Drawing for the job (mm, zero at the part's lowest x, y, z). A direction names the side the tool comes from. Coordinates: 2 decimals unless noted, no trailing zeros. Loops run counter-clockwise (first coordinate to the right, second up) from the corner with the lowest first, then second, coordinate; pieces in that order, holes last. Notation, with made-up numbers: (53, 24) -> (79, 24) arc R16 ccw to (79, 42) -> close; hole circle Ø9 at (-32, 68). An arc over 180 degrees is marked (long way). Write each question's results on one line, items separated by ' | '.
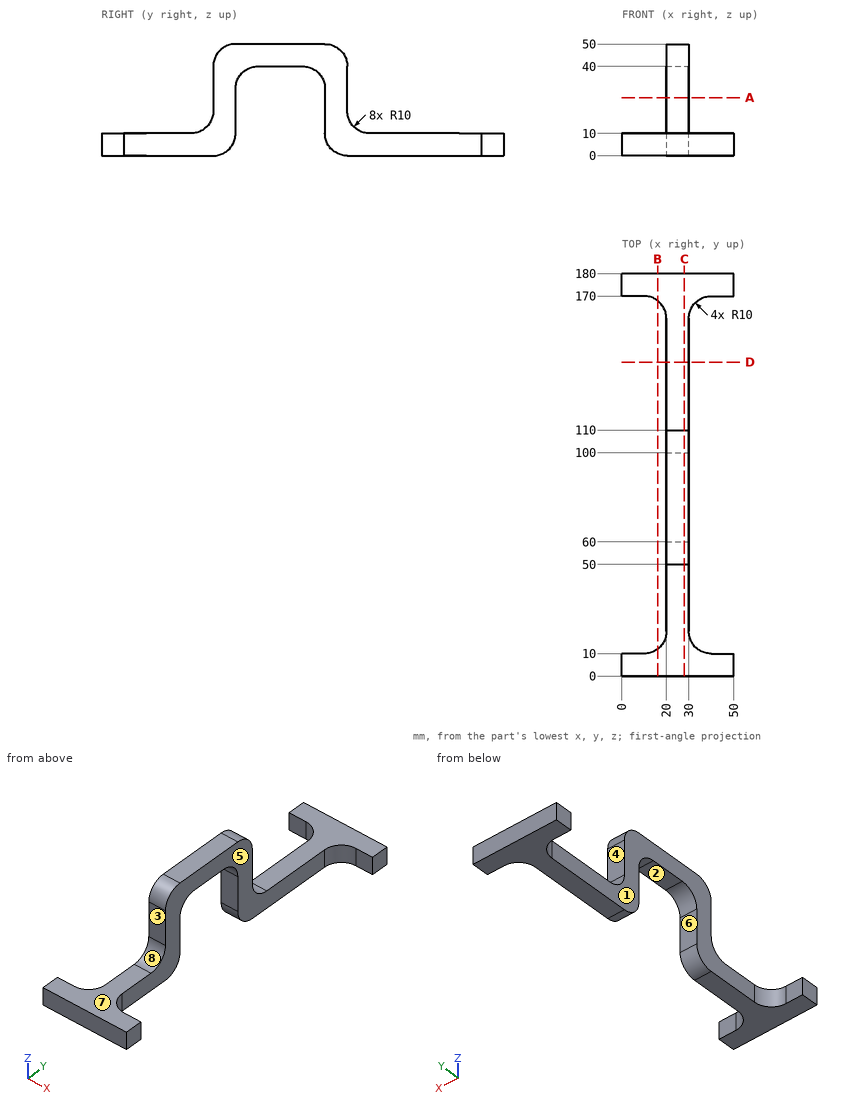
1) Slice it at C-C (x = 28). Write the cut outline in (y, z), then the cut area to 3 significant figures.
Outcome:
outline: (0, 0) -> (50, 0) arc R10 ccw to (60, 10) -> (60, 30) arc R10 cw to (70, 40) -> (90, 40) arc R10 cw to (100, 30) -> (100, 10) arc R10 ccw to (110, 0) -> (180, 0) -> (180, 10) -> (120, 10) arc R10 cw to (110, 20) -> (110, 40) arc R10 ccw to (100, 50) -> (60, 50) arc R10 ccw to (50, 40) -> (50, 20) arc R10 cw to (40, 10) -> (0, 10) -> close | area: 2,600 mm^2
2) Two-plate mould, pull along Y, no slides. Class the marked faces 6, 7 and 8: pulls with the +Y half, pulls with the -Y half, needs draft (parallel to the pull), parting line crosses it, or undercut.
Outcome:
face 6: undercut | face 7: needs draft | face 8: pulls with the -Y half
3) Drill centre lines: L1, parallel to Y at x = 23, z = 20; L2, parallel to X at y = 51.5, z = 32; L3, parallel to Y at x = 17, z = 4. Where is each one in solid material? Low to high. Write a range as from..to.
Outcome:
L1: y = 50..60, 100..110 | L2: x = 20..30 | L3: y = 0..12.86, 167.14..180
4) Pin check, flat tips, straight feed: pin 1 (12 mm diameter, centred on y = 48.5, z = 42, fed in from -X); pin 2 (25 mm diameter, centred on x = 36.5, y = 140.5, fed in from +Z); pin 3 (4 mm diameter, centred on x = 26, y = 109, fed in from -Z); pin 4 (3 mm diameter, centred on x = 23.5, z = 25, fed in from +Y). Stop position of each tip, or through.
Outcome:
pin 1: stops at x = 20 | pin 2: stops at z = 10 | pin 3: stops at z = 0 | pin 4: stops at y = 110
5) Which spindle directions (+Z, -Z, +X, -X, +Y, -Y) get a long thin tool onto all of the face, cutting with end or side? Do the marked faces 1, 2, 3, 4 and 5. Say none if no direction does.
Outcome:
face 1: +Z, -Z, -X | face 2: -Z, +X, -X | face 3: +Z, +X, -X, -Y | face 4: +Z, +X, -X, +Y | face 5: +Z, -Z, +X
6) Slice it at B-B (x = 16). Write the cut outline in (y, z).
Outcome:
outline: (0, 0) -> (12, 0) -> (12, 10) -> (0, 10) -> close; (168, 0) -> (180, 0) -> (180, 10) -> (168, 10) -> close
7) Slice it at D-D (y = 140.5). Write the cut outline in (x, z).
Outcome:
outline: (20, 0) -> (30, 0) -> (30, 10) -> (20, 10) -> close
8) Slice it at A-A (z = 26). Write the cut outline in (x, y), then the cut area to 3 significant figures.
Outcome:
outline: (20, 50) -> (30, 50) -> (30, 60) -> (20, 60) -> close; (20, 100) -> (30, 100) -> (30, 110) -> (20, 110) -> close | area: 200 mm^2
